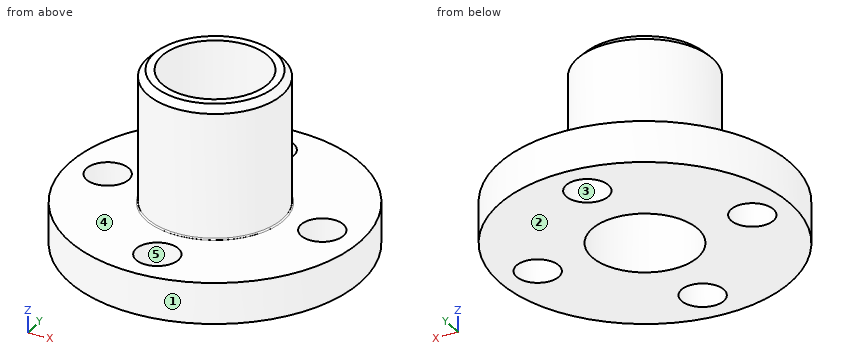
```python
from build123d import *

# Parameters (mm, degrees)
SKETCH1_R                = 11
SKETCH1_R_2              = 5.075
BOSS_EXTRUDE1_DEPTH      = 3.1
BOSS_EXTRUDE2_DEPTH      = 10
BOSS_EXTRUDE2_DEPTH_BACK = 3.1
SKETCH2_R                = 5.1
SKETCH2_R_2              = 4
CHAMFER1_SIZE            = 0.5
FILLET1_R                = 0.1
SKETCH3_R                = 1.6
CUT_EXTRUDE1_DEPTH       = 10


with BuildPart() as part:
    # Sketch1 → Boss-Extrude1 (new body)
    with BuildSketch(Plane.XY):
        with Locations(Location((0, 0, 0), (0, 0, 180))):
            Circle(SKETCH1_R)
        with Locations(Location((0, 0, 0), (0, 0, 180))):
            Circle(SKETCH1_R_2, mode=Mode.SUBTRACT)
    extrude(amount=BOSS_EXTRUDE1_DEPTH)

    # Sketch2 → Boss-Extrude2 (add, two sides: drawn at the far end of the back side and taken through both)
    with BuildSketch(Plane.XY.offset(3.1).offset(-BOSS_EXTRUDE2_DEPTH_BACK)):
        Circle(SKETCH2_R)
        Circle(SKETCH2_R_2, mode=Mode.SUBTRACT)
    extrude(amount=BOSS_EXTRUDE2_DEPTH + BOSS_EXTRUDE2_DEPTH_BACK)

    # Chamfer1
    chamfer1_edges = [part.edges().sort_by_distance(p)[0] for p in [
        (-5.1, 0, 13.1),
    ]]
    chamfer(chamfer1_edges, length=CHAMFER1_SIZE)

    # Fillet1
    fillet1_edges = [part.edges().sort_by_distance(p)[0] for p in [
        (-5.1, 0, 3.1),
    ]]
    fillet(fillet1_edges, radius=FILLET1_R)

    # Sketch3 → Cut-Extrude1 (cut)
    with BuildSketch(Plane.XY.offset(3.1)):
        with Locations((0, 8.05)):
            Circle(SKETCH3_R)
        with Locations((8.05, 0)):
            Circle(SKETCH3_R)
        with Locations((0, -8.05)):
            Circle(SKETCH3_R)
        with Locations((-8.05, 0)):
            Circle(SKETCH3_R)
    extrude(amount=-CUT_EXTRUDE1_DEPTH, mode=Mode.SUBTRACT)


solid = part.part
```
Source: CAD feature listing. Evaluate the final solid. Frame: model axes, mm. Face numbers are marked on the shaded views. A direction names the side the tool comes from. Coordinates: 2 decimals unless noted, no trailing zeros. Loops run counter-clockwise (first coordinate to the right, second up) from the corner with the lowest first, then second, coordinate; pieces in that order, holes last. Notation, with made-up numbers: M 6.25,84.5 L 34.25,84.5 A21 cw 34.25,90.5 Z; hole C -4,27 d10. An arc over 180 degrees is marked long. Use a Markdown table: item, result. Add a question column.
Q1. Draft query along X for the marked faces 1, 2 and 3. Return one class per face: pulls with the +X half, pulls with the -X half, needs draft (parallel to the pull), parting line crosses it, or undercut.
Q2. Access query for the marked faces 4 and 5. Directions: +Z, -Z, +X, -X, +Y, -Y. A direction counts if a zero-diameter tool reaches every point of the face in a straight line with its end or side. Return the directions, or none.
Q3. Section query D-D, the plane y = -8.05. Return loops of the section in (x, z).
Q4. Section query C-C, the plane x = 8. Return loops of the section in (y, z).
Q5. Material intervals for L1, parallel to Y at x = 0, z = 1.2; L2, parallel to X at y = 0.25, z = 1; L3, parallel to Z at x = 4.5, y = 3.75, sorted ascending.
Q6. First-contact query: pin 1 (5 mm diameter, centred on x = -3, y = -8, fed in from +Z); pin 2 (8 mm diameter, centred on x = -3.5, y = -8, fed in from +Z); pin 3 (6 mm diameter, centred on x = 4, z = 8.5, fed in from +Y). Flat tips, straight axial feed; report the tip coordinate or a pass-through.
Q7. Section query A-A, the plane x = 0. Return loops of the section in (y, z).
Result:
| question | item | result |
|---|---|---|
| 1 | face 1 | parting line crosses it |
| 1 | face 2 | needs draft |
| 1 | face 3 | undercut |
| 2 | face 4 | +Z |
| 2 | face 5 | +Z, -Z |
| 3 | outline | M -7.5,0 L -1.6,0 L -1.6,3.1 L -7.5,3.1 Z; M 1.6,0 L 7.5,0 L 7.5,3.1 L 1.6,3.1 Z |
| 4 | outline | M -7.55,0 L -1.6,0 L -1.6,3.1 L -7.55,3.1 Z; M 1.6,0 L 7.55,0 L 7.55,3.1 L 1.6,3.1 Z |
| 5 | L1 | y = -11 to -9.65, -6.45 to -4, 4 to 6.45, 9.65 to 11 |
| 5 | L2 | x = -11 to -9.63, -6.47 to -3.99, 3.99 to 6.47, 9.63 to 11 |
| 5 | L3 | z = 0 to 3.1 |
| 6 | pin 1 | stops at z = 3.1 |
| 6 | pin 2 | stops at z = 12.97 |
| 6 | pin 3 | stops at y = 5 |
| 7 | outline | M -11,0 L -9.65,0 L -9.65,3.1 L -11,3.1 Z; M -6.45,0 L -4,0 L -4,13.1 L -4.6,13.1 L -5.1,12.6 L -5.1,3.2 A0.1 cw -5.2,3.1 L -6.45,3.1 Z; M 4,0 L 6.45,0 L 6.45,3.1 L 5.2,3.1 A0.1 cw 5.1,3.2 L 5.1,12.6 L 4.6,13.1 L 4,13.1 Z; M 9.65,0 L 11,0 L 11,3.1 L 9.65,3.1 Z |
